Part model, mm, in its own coordinate system. Face numbers are marked on the shaded views. A direction names the side the tool comes from. Round coordinates to 2 decimals unless told otherwise and drop trailing zeros. Loops run counter-clockwise (first coordinate to the right, second up) from the corner with the lowest first, then second, coordinate; pieces in that order, holes last. Notation, with made-up numbers: (-20.5, 58) - (7.5, 58) arc R21 cw to (7.5, 87) - close; hole circle Ø5 at (-3, 26). An arc over 180 degrees is marked (long way). Put each result on its own line as item: value.
from build123d import *

# Parameters (mm, degrees)
SKETCH1_W                                        = 32
SKETCH1_H                                        = 65
BOSS_EXTRUDE1_DEPTH                              = 7
TAP_DRILL_FOR_M3X0_5_TAP1_D                      = 2.5
CBORE_FOR_1_4_SOCKET_HEAD_CAP_SCREW1_D           = 6.7564
CBORE_FOR_1_4_SOCKET_HEAD_CAP_SCREW1_CBORE_D     = 11.1125
CBORE_FOR_1_4_SOCKET_HEAD_CAP_SCREW1_CBORE_DEPTH = 6.35
SKETCH6_W                                        = 11.1125
SKETCH6_H                                        = 25.4
CUT_EXTRUDE1_DEPTH                               = 6.35
SKETCH7_W                                        = 6.7564
SKETCH7_H                                        = 25.4
CUT_EXTRUDE2_DEPTH                               = 87.167337251


with BuildPart() as part:
    # Sketch1 → Boss-Extrude1 (new body)
    with BuildSketch(Plane.XZ.offset(-27.928124556)):
        with Locations((22.96435644, 44.091555907)):
            Rectangle(SKETCH1_W, SKETCH1_H)
    extrude(amount=BOSS_EXTRUDE1_DEPTH)

    # Tap Drill for M3x0.5 Tap1 (through all)
    with Locations(Plane(origin=(0, 27.928124556, 0), x_dir=(1, 0, 0), z_dir=(0, 1, 0))):
        with Locations((10.96435606, -15.591555987), (34.96435632, -15.591555987), (34.96435632, -72.591556287), (10.96435606, -72.591556287)):
            Hole(TAP_DRILL_FOR_M3X0_5_TAP1_D / 2)

    # CBORE for 1/4 Socket Head Cap Screw1 (through all)
    with Locations(Plane(origin=(0, 27.928124556, 0), x_dir=(1, 0, 0), z_dir=(0, 1, 0))):
        with Locations((22.96435644, -31.391555907), (22.96435644, -56.791555907)):
            CounterBoreHole(CBORE_FOR_1_4_SOCKET_HEAD_CAP_SCREW1_D / 2, CBORE_FOR_1_4_SOCKET_HEAD_CAP_SCREW1_CBORE_D / 2, CBORE_FOR_1_4_SOCKET_HEAD_CAP_SCREW1_CBORE_DEPTH)

    # Sketch6 → Cut-Extrude1 (cut)
    with BuildSketch(Plane(origin=(0, 27.928124556, 0), x_dir=(1, 0, 0), z_dir=(0, 1, 0))):
        with Locations((22.96435644, -44.091555907)):
            Rectangle(SKETCH6_W, SKETCH6_H)
    extrude(amount=-CUT_EXTRUDE1_DEPTH, mode=Mode.SUBTRACT)

    # Sketch7 → Cut-Extrude2 (cut, through all)
    with BuildSketch(Plane(origin=(0, 21.578124556, 0), x_dir=(1, 0, 0), z_dir=(0, 1, 0))):
        with Locations((22.96435644, -44.091555907)):
            Rectangle(SKETCH7_W, SKETCH7_H)
    extrude(amount=-CUT_EXTRUDE2_DEPTH, mode=Mode.SUBTRACT)


solid = part.part
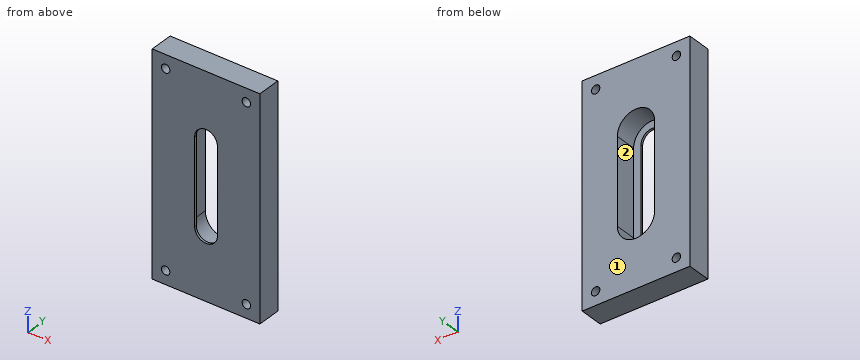
1. Probe line 1 along X through (y, z) = (27, 33.5); line 2 along Z through (x, y) = (12, 22.5); line 3 along Z through (x, y) = (11.5, 23.5). List the from-to ranges inside material, lowest first. Write a range as [from, to].
A:
line 1: x = [6.96, 17.41], [28.52, 38.96]
line 2: z = [11.59, 14.89], [16.29, 71.89], [73.29, 76.59]
line 3: z = [11.59, 14.46], [16.72, 71.46], [73.72, 76.59]
2. Band-saw the part on D-D (x = 23). List the corners of the cut face in (y, z).
A:
outline: (20.93, 11.59) - (27.93, 11.59) - (27.93, 25.84) - (21.58, 25.84) - (21.58, 28.01) - (20.93, 28.01) - close; (20.93, 60.17) - (21.58, 60.17) - (21.58, 62.35) - (27.93, 62.35) - (27.93, 76.59) - (20.93, 76.59) - close
3. Band-saw the part on B-B (x = 35). List the corners of the cut face in (y, z).
A:
outline: (20.93, 11.59) - (27.93, 11.59) - (27.93, 14.34) - (20.93, 14.34) - close; (20.93, 16.84) - (27.93, 16.84) - (27.93, 71.34) - (20.93, 71.34) - close; (20.93, 73.84) - (27.93, 73.84) - (27.93, 76.59) - (20.93, 76.59) - close
4. Tool access for the marked faces 1 and 2: list every direction of +Z, -Z, +X, -X, +Y, -Y with a clear straight run to the whole face (end or side of a thin tool).
A:
face 1: +Z, -Z, +X, -X, +Y
face 2: +Y
5. Band-saw the part on C-C (y = 23). List the corners of the cut face in (x, z).
A:
outline: (6.96, 11.59) - (38.96, 11.59) - (38.96, 76.59) - (6.96, 76.59) - close; hole circle Ø2.5 at (10.96, 15.59); hole circle Ø2.5 at (10.96, 72.59); hole (17.41, 31.39) arc R5.56 ccw to (28.52, 31.39) - (28.52, 56.79) arc R5.56 ccw to (17.41, 56.79) - close; hole circle Ø2.5 at (34.96, 15.59); hole circle Ø2.5 at (34.96, 72.59)
6. Band-saw the part on A-A (z = 38). List the corners of the cut face in (x, y).
A:
outline: (6.96, 20.93) - (19.59, 20.93) - (19.59, 21.58) - (17.41, 21.58) - (17.41, 27.93) - (6.96, 27.93) - close; (26.34, 20.93) - (38.96, 20.93) - (38.96, 27.93) - (28.52, 27.93) - (28.52, 21.58) - (26.34, 21.58) - close
